Geometry: final body of the model. Coordinates: model frame, mm. A direction names the side the tool comes from. Give positions to 0.01 mm unless a question says otherwise; leave off trailing zeros. Write each loop counter-clockwise with the first axis right and the second up, starting at its lowest first coordinate (ties: lowest second). Pieces come first, ordered by that corner, then holes. Notation, with made-up numbers: (70, -6) - (105, -6) arc R36 cw to (105, 28) - close; hole circle Ø3 at (-9, 9). An arc over 180 degrees is marked (long way). Use CSV: the item, a comma, the result in double quotes. Start each with the question number.
(1) Reachability of faces 1 (the flat face through (2, -35, 15)), 2 (the cylindrical face through (2, -6.4, 35.6)) from +Z, -Z, +X, -X, +Y, -Y: full face, straight path, thin tool, end or side. Return the list, or none.
(2) Section A-A on x = 3.4. Output: boundary loops of the cut face in (y, z), and give its area (3 significant figures).
(3) Section D-D on y = -6.5. Output: boundary loops of the cut face in (x, z).
(4) Section C-C on z = 0. Output: boundary loops of the cut face in (x, y), and give its area (3 significant figures).
(5) Draft query along Z for faces 3 (the cylindrical face through (2.028, -4.34, 14.985)), 4 (the flat face through (2, 0, 40)), 5 (the flat face through (2, -35, -15)). Return one class per face: released by +Z, released by -Z, zero draft, split by the parting line, or undercut.
(6) Line query: probe 1 along Y at (x, z) = (3.05, 0); probe 2 along Y at (x, z) = (1.85, -2); probe 3 along Z at (x, y) = (1.85, -46). Output: solid intervals per line, ascending. Write a range as [from, to].
(7) Section B-B on z = 11. Output: boundary loops of the cut face in (x, y), and give its area (3 significant figures).
(8) First-contact query: pin 1 Ø4 at (y, z) = (-6.5, -33) entering from +X; pin 2 Ø1.2 at (x, y) = (1.5, -39.5) entering from -Z; pin 3 Ø2 at (x, z) = (2, 25.5) entering from -Y. Flat tips, straight axial feed; report the tip coordinate or a pass-through.
from build123d import *

# Parameters (mm, degrees)
BOSS_EXTRUDE1_DEPTH = 4
SKETCH2_R           = 15
SKETCH2_R_2         = 2.6
CUT_EXTRUDE1_DEPTH  = 5
FILLET1_R           = 10


with BuildPart() as part:
    # Sketch1 → Boss-Extrude1 (new body)
    with BuildSketch(Plane(origin=(0, 0, 0), x_dir=(0, 0, -1), z_dir=(1, 0, 0))):
        Polygon((-40, -15), (-15, -15), (-15, -55), (15, -55), (15, -15), (40, -15), (40, 15), (-40, 15), align=None)
    extrude(amount=BOSS_EXTRUDE1_DEPTH)

    # Sketch2 → Cut-Extrude1 (cut)
    with BuildSketch(Plane(origin=(4, 0, 0), x_dir=(0, 0, -1), z_dir=(1, 0, 0))):
        with Locations((0, -5)):
            Circle(SKETCH2_R)
        with Locations((0, -45)):
            Circle(SKETCH2_R_2)
        with Locations((-33, -6.5)):
            Circle(SKETCH2_R_2)
        with Locations((33, -6.5)):
            Circle(SKETCH2_R_2)
    extrude(amount=-CUT_EXTRUDE1_DEPTH, mode=Mode.SUBTRACT)

    # Fillet1
    fillet1_edges = [part.edges().sort_by_distance(p)[0] for p in [
        (2, 15, 40),
        (2, 15, -40),
        (2, -15, -40),
        (2, -15, -15),
        (2, -55, -15),
        (2, -55, 15),
        (2, -15, 15),
        (2, -15, 40),
    ]]
    fillet(fillet1_edges, radius=FILLET1_R)


solid = part.part
Check values:
1,face 1,"+Z, +X, -X, -Y"
1,face 2,"+X, -X"
2,outline,"(-55, -5) arc R10 ccw to (-45, -15) - (-25, -15) arc R10 cw to (-15, -25) - (-15, -30) arc R10 ccw to (-5, -40) - (5, -40) arc R10 ccw to (15, -30) - (15, 30) arc R10 ccw to (5, 40) - (-5, 40) arc R10 ccw to (-15, 30) - (-15, 25) arc R10 cw to (-25, 15) - (-45, 15) arc R10 ccw to (-55, 5) - close; hole circle Ø5.2 at (-45, 0); hole circle Ø30 at (-5, 0); hole circle Ø5.2 at (-6.5, -33); hole circle Ø5.2 at (-6.5, 33)"
2,area,"2,740 mm²"
3,outline,"(0, -39.89) - (4, -39.89) - (4, -35.6) - (0, -35.6) - close; (0, -30.4) - (4, -30.4) - (4, -14.92) - (0, -14.92) - close; (0, 14.92) - (4, 14.92) - (4, 30.4) - (0, 30.4) - close; (0, 35.6) - (4, 35.6) - (4, 39.89) - (0, 39.89) - close"
4,outline,"(0, -55) - (4, -55) - (4, -47.6) - (0, -47.6) - close; (0, -42.4) - (4, -42.4) - (4, -20) - (0, -20) - close; (0, 10) - (4, 10) - (4, 15) - (0, 15) - close"
4,area,"139 mm²"
5,face 3,"undercut"
5,face 4,"released by +Z"
5,face 5,"released by -Z"
6,probe 1,"y = [-55, -47.6], [-42.4, -20], [10, 15]"
6,probe 2,"y = [-55, -46.66], [-43.34, -19.87], [9.87, 15]"
6,probe 3,"z = [-14.95, -2.4], [2.4, 14.95]"
7,outline,"(0, -53) - (4, -53) - (4, -15.2) - (0, -15.2) - close; (0, 5.2) - (4, 5.2) - (4, 15) - (0, 15) - close"
7,area,"190 mm²"
8,pin 1,"passes through"
8,pin 2,"stops at z = -15"
8,pin 3,"stops at y = -15.01"
